Work out the finished part from the listing and answer in its coordinate system (mm). A direction names the side the tool comes from. Round coordinates to 2 decimals unless told otherwise and drop trailing zeros. Write each loop counter-clockwise with the first axis right and the second up, starting at its lowest first coordinate (ties: lowest second). Pieces come first, ordered by that corner, then holes.
1. Flat-ended cylindrical pins translate along their axes: pin 1 Ø2.5 at (x, y) = (-24.09, 9.2) entering from -Z (1 decimal); pin 2 Ø4 at (x, y) = (-4.45, 10) entering from +Z; pin 3 Ø1 at (y, z) = (-1, 2.5) entering from +X; pin 4 Ø2 at (x, z) = (10.11, 2.41) entering from +Y. Find the tip coordinate at first contact, or state that the pin passes through.
2. Straight lines are drawn through the part: probe 1 along X at (y, z) = (10.5, 3.5); probe 2 along X at (y, z) = (7.5, 4); probe 3 along Y at (x, z) = (-20, 1.95). For each, find the intervals that lie inside material, in ascending order.
3. Find section B-B (y = 9.2). Write down the section's boundary in (x, z), and give its area (3 significant figures).
4. Find section A-A (z = 0.5). Write down the section's boundary in (x, y), and give its area (3 significant figures).
5. Determine the mould class of faces 1 (the face through (-8, 7, 0)), 2 (the face through (6.428, 11.606, 2.379)), 3 (the face through (-22.183, 9.801, 2.379)), 4 (the face through (-4.28, 11.24, 2.38)) for opening direction Y: pulls with the +Y half, pulls with the -Y half, needs draft (parallel to the pull), parting line crosses it, or undercut.
6. Find section C-C (x = -24). Write down the section's boundary in (y, z).
7. A tool of negligible diameter and unlimited length cuts with its end or side. For faces 5 (the face through (-17.391, -1, 2)), 6 (the face through (-2.65, 2.54, 1.42)), 7 (the face through (-20.054, 7.24, 2.379)), from which of +Z, -Z, +X, -X, +Y, -Y can it reach the whole face along a straight path? Write none if from no direction.
8. Find section D-D (y = 12.5). Write down the section's boundary in (x, z), and give its area (3 significant figures).
```python
from build123d import *

# Parameters (mm, degrees)
BOSS_EXTRUDE1_DEPTH             = 4.826
M3X0_5_TAPPED_HOLE1_D           = 2.5
TAP_DRILL_FOR_M3X0_5_TAP1_D     = 2.5
TAP_DRILL_FOR_M3X0_5_TAP1_DEPTH = 5
TAP_DRILL_FOR_M3X0_5_TAP1_TIP   = 0.751075774
SKETCH1_3_R                     = 2
BOSS_EXTRUDE2_DEPTH             = 4.826
M3X0_5_TAPPED_HOLE2_D           = 2.5
FILLET1_R                       = 1
M2_TAPPED_HOLES_D               = 1.6
FILLET2_R                       = 0.5


with BuildPart() as part:
    # Sketch1 → Boss-Extrude1 (new body)
    with BuildSketch(Plane.XY):
        Polygon((13.109289519, 0), (0, 0), (-8.890710481, 0), (-8.890710481, 17), (0, 17), (13.109289519, 6), align=None)
    extrude(amount=BOSS_EXTRUDE1_DEPTH)

    # M3x0.5 Tapped Hole1 (through all)
    with Locations(Plane.XY.offset(4.826)):
        with Locations((-4.445355241, 10)):
            Hole(M3X0_5_TAPPED_HOLE1_D / 2)

    # Tap Drill for M3x0.5 Tap1
    with Locations(Plane(origin=(-1.890710481, 0, 2.413), x_dir=(0, 0, -1), z_dir=(0, -1, 0))):
        with Locations((0, 0), (0, 12)):
            Hole(TAP_DRILL_FOR_M3X0_5_TAP1_D / 2, depth=TAP_DRILL_FOR_M3X0_5_TAP1_DEPTH)
            with Locations((0, 0, -(TAP_DRILL_FOR_M3X0_5_TAP1_DEPTH + TAP_DRILL_FOR_M3X0_5_TAP1_TIP / 2))):  # 118° drill point
                Cone(0, TAP_DRILL_FOR_M3X0_5_TAP1_D / 2, TAP_DRILL_FOR_M3X0_5_TAP1_TIP, mode=Mode.SUBTRACT)

    # Sketch1<3> → Boss-Extrude2 (add)
    with BuildSketch(Plane.XY):
        Polygon((-17.390710481, 0), (-8.890710481, 0), (-8.890710481, 17), (-17.390710481, 17), (-28.890710481, 17), (-28.890710481, -3.3), (-17.390710481, -3.3), align=None)
        with Locations((-24.090710481, 9.2)):
            Circle(SKETCH1_3_R, mode=Mode.SUBTRACT)
    extrude(amount=BOSS_EXTRUDE2_DEPTH)

    # M3x0.5 Tapped Hole2 (through all)
    with Locations(Plane.XY.offset(4.826)):
        with Locations((-4.390710481, 14.5)):
            Hole(M3X0_5_TAPPED_HOLE2_D / 2)

    # Fillet1
    fillet1_edges = [part.edges().sort_by_distance(p)[0] for p in [
        (0, 17, 2.413),
        (13.109289519, 6, 2.413),
        (-28.890710481, 17, 2.413),
        (-28.890710481, -3.3, 2.413),
        (-17.390710481, -3.3, 2.413),
    ]]
    fillet(fillet1_edges, radius=FILLET1_R)

    # M2 Tapped Holes (through all)
    with Locations(Plane.XY.offset(4.826)):
        with Locations((-19.290710481, 12.5), (-19.290710481, 7)):
            Hole(M2_TAPPED_HOLES_D / 2)

    # Fillet2
    fillet2_edges = [part.edges().sort_by_distance(p)[0] for p in [
        (-17.390710481, 0, 2.413),
    ]]
    fillet(fillet2_edges, radius=FILLET2_R)


solid = part.part
```
Worked answers:
1. pin 1: passes through
1. pin 2: stops at z = 4.83
1. pin 3: stops at x = -17.39
1. pin 4: stops at y = 9.36
2. probe 1: x = -28.89 to -25.61, -22.57 to -5.59, -3.3 to 7.75
2. probe 2: x = -28.89 to -25.14, -23.04 to -19.92, -18.67 to 11.32
2. probe 3: y = -3.3 to 6.63, 7.37 to 12.13, 12.87 to 17
3. outline: (-28.89, 0) - (-26.09, 0) - (-26.09, 4.83) - (-28.89, 4.83) - close; (-22.09, 0) - (-5.41, 0) - (-5.41, 4.83) - (-22.09, 4.83) - close; (-3.48, 0) - (9.3, 0) - (9.3, 4.83) - (-3.48, 4.83) - close
3. area: 156 mm2
4. outline: (-28.89, -2.3) arc R1 ccw to (-27.89, -3.3) - (-18.39, -3.3) arc R1 ccw to (-17.39, -2.3) - (-17.39, -0.5) arc R0.5 cw to (-16.89, 0) - (13.11, 0) - (13.11, 5.53) arc R1 ccw to (12.75, 6.3) - (0.28, 16.77) arc R1 ccw to (-0.36, 17) - (-27.89, 17) arc R1 ccw to (-28.89, 16) - close; hole circle Ø4 at (-24.09, 9.2); hole circle Ø1.6 at (-19.29, 7); hole circle Ø1.6 at (-19.29, 12.5); hole circle Ø2.5 at (-4.45, 10); hole circle Ø2.5 at (-4.39, 14.5)
4. area: 653 mm2
5. face 1: needs draft
5. face 2: pulls with the +Y half
5. face 3: undercut
5. face 4: undercut
6. outline: (-3.3, 0) - (7.2, 0) - (7.2, 4.83) - (-3.3, 4.83) - close; (11.2, 0) - (17, 0) - (17, 4.83) - (11.2, 4.83) - close
7. face 5: +Z, -Z, +X, -Y
7. face 6: -Y
7. face 7: +Z, -Z
8. outline: (-28.89, 0) - (-20.09, 0) - (-20.09, 4.83) - (-28.89, 4.83) - close; (-18.49, 0) - (5.36, 0) - (5.36, 4.83) - (-18.49, 4.83) - close
8. area: 158 mm2
